Autodesk Inventor part; units mm, degrees
ref_plane "YZ Plane" through (0, 0, 0) normal (1, 0, 0) x (0, 1, 0)
ref_plane "XZ Plane" through (0, 0, 0) normal (0, 1, 0) x (-1, 0, 0)
ref_plane "XY Plane" through (0, 0, 0) normal (0, 0, 1) x (1, 0, 0)
sketch "Sketch1" plane through (0, 0, 0) normal (0, 0, 1) x (1, 0, 0)
  circle A0 centre (0, 0) radius 7.5
  circle A1 centre (0, 63) radius 5
  circle A2 centre (0, 0) radius 15
  circle A3 centre (0, 63) radius 10
  line L0 (-9.9685, 63.7937) -> (-14.9527, 1.1905)
  line L1 (9.9685, 63.7937) -> (14.9527, 1.1905)
  dimension "d0" = 63
  dimension "d1" = 30
  dimension "d2" = 20
  dimension "d3" = 10
  dimension "d4" = 15
extrude "Extrusion1" add sketch "Sketch1" along normal mid plane 10
properties part number "Eslabón 2" material "Stainless Steel"
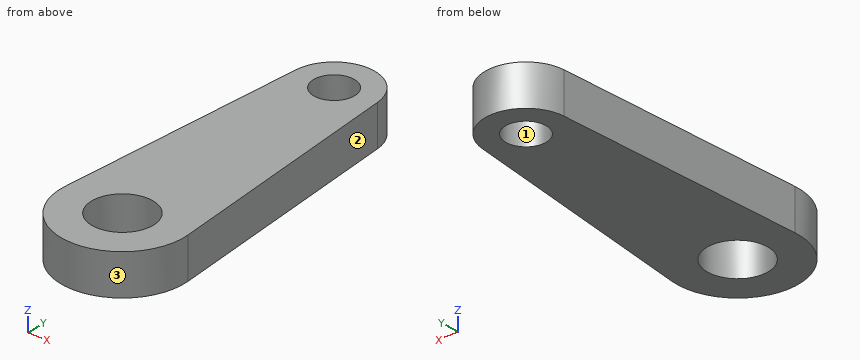
Geometry: final body of the model. Coordinates: model frame, mm. Face numbers are marked on the shaded views. Round coordinates to 2 decimals unless told otherwise and drop trailing zeros. Order: outer loops, then holes, each group sorted by start corner. A loop starts at its lowest first (then second) coordinate and runs counter-clockwise, first axis right, second up. Notation, with made-up numbers: (0.25, 14.25) - (32.25, 14.25) arc R28 ccw to (32.25, 46.25) - close; hole circle Ø11 at (83.5, 9). An arc over 180 degrees is marked (long way). Write each question's results on one line, items separated by ' | '.
Item 1: Section D-D, the plane y = 63. Return the cut outline in (x, z), and give its area (3 significant figures).
Completed:
outline: (-10.03, -5) - (-5, -5) - (-5, 5) - (-10.03, 5) - close; (5, -5) - (10.03, -5) - (10.03, 5) - (5, 5) - close | area: 101 mm^2
Item 2: Section B-B, the plane x = 0. Return the cut outline in (y, z).
Completed:
outline: (-15, -5) - (-7.5, -5) - (-7.5, 5) - (-15, 5) - close; (7.5, -5) - (58, -5) - (58, 5) - (7.5, 5) - close; (68, -5) - (73, -5) - (73, 5) - (68, 5) - close
Item 3: Mould query, pull axis X, two halves, no side actions, for the marked faces 1, 2 and 3. Classes: pulls with the +X half, pulls with the -X half, needs draft (parallel to the pull), parting line crosses it, or undercut.
Completed:
face 1: undercut | face 2: pulls with the +X half | face 3: parting line crosses it
Item 4: First-contact query: pin 1 Ø3 at (y, z) = (4.5, 4) entering from -X; pin 2 Ø3 at (x, z) = (5, 3) entering from -Y; pin 3 Ø4 at (x, z) = (11, -0.5) entering from -Y. Flat tips, straight axial feed; report the tip coordinate or a pass-through.
Completed:
pin 1: x = -14.81 | pin 2: y = -14.59 | pin 3: y = -12
Item 5: Section A-A, the plane y = 0. Return the cut outline in (x, z), and give its area (3 significant figures).
Completed:
outline: (-15, -5) - (-7.5, -5) - (-7.5, 5) - (-15, 5) - close; (7.5, -5) - (15, -5) - (15, 5) - (7.5, 5) - close | area: 150 mm^2
Item 6: Material intervals for line 1 along Y through (x, z) = (-1.5, -3.25); line 2 along Y through (x, z) = (-4, -2.75); line 3 along Y through (x, z) = (-6.5, -4.5), sorted ascending. Write a range as [from, to].
Completed:
line 1: [-14.92, -7.35], [7.35, 58.23], [67.77, 72.89] | line 2: [-14.46, -6.34], [6.34, 60], [66, 72.17] | line 3: [-13.52, -3.74], [3.74, 70.6]
Item 7: Section C-C, the plane z = -4. Return the cut outline in (x, y).
Completed:
outline: (-14.95, 1.19) arc R15 ccw (long way) to (14.95, 1.19) - (9.97, 63.79) arc R10 ccw to (-9.97, 63.79) - close; hole circle Ø15 at (0, 0); hole circle Ø10 at (0, 63)
